Geometry check sheet. Reference: the model listing, model coordinates, mm. Coordinates: 2 decimals unless noted, no trailing zeros. Loops run counter-clockwise (first coordinate to the right, second up) from the corner with the lowest first, then second, coordinate; pieces in that order, holes last. Notation, with made-up numbers: (83, -25) -> (138, -25) arc R19 cw to (138, -14) -> close; hole circle Ø1 at (-23.5, 28). An arc over 180 degrees is marked (long way). Answer as a JSON object with one key per item and string values.
from build123d import *

# Parameters (mm, degrees)
F0_R     = 8
F1_DEPTH = 6
F4_DEPTH = 16.001
F5_R     = 20
F6_R     = 0.5


with BuildPart() as f1:
    # F0 (on Top) → F1 (new body)
    with BuildSketch(Plane.XY):
        Circle(F0_R)
    extrude(amount=F1_DEPTH)

    # F3 (on offset) → F4 (cut, through all)
    with BuildSketch(Plane.XZ.offset(8)):
        Polygon((8, 6), (-8, 6), (0, 4.4), align=None)
    extrude(amount=-F4_DEPTH, mode=Mode.SUBTRACT)

    # F5
    f5_edges = [f1.edges().sort_by_distance(p)[0] for p in [
        (0, 0, 4.4),
    ]]
    fillet(f5_edges, radius=F5_R)

    # F6
    f6_edges = [f1.edges().sort_by_distance(p)[0] for p in [
        (-6.896857, -4.053808, 5.779371),
        (-6.896857, 4.053808, 5.779371),
    ]]
    fillet(f6_edges, radius=F6_R)


solid = f1.part
1. Mould release check, pull along X, two halves, no side actions. Record for faces 1 (the face through (3.69, -7.1, 2.66)), 2 (the face through (-5.3, -0.09, 5.46)), 3 (the face through (0, 0, 0)): released by +X, released by -X, zero draft, split by the parting line, or undercut.
Evaluation:
{"face 1": "split by the parting line", "face 2": "undercut", "face 3": "zero draft"}
2. Depth check by flat-ended pin: P1, Ø1, axis at y = 3.5, z = 2, coming from the -X side; P2, Ø1.5, axis at x = -4.5, y = -3, coming from the -Z side; P3, Ø3, axis at x = -4.5, y = 2, coming from the +Z side; P4, Ø6, axis at x = -1, y = -3.5, coming from the +Z side. Enter the tip coordinate at first touch or a pass-through.
Evaluation:
{"P1": "stops at x = -7.42", "P2": "stops at z = 0", "P3": "stops at z = 5.6", "P4": "stops at z = 5.2"}
3. Thickness scan on probe 1 along X at (y, z) = (0.25, 2.3); probe 2 along Z at (x, y) = (3, 6); probe 3 along X at (y, z) = (7.25, 3.9). Record the ranges inside material, lowest first. Write a range as from..to.
Evaluation:
{"probe 1": "x = -8..8", "probe 2": "z = 0..5.02", "probe 3": "x = -3.38..3.38"}
4. Section check A-A, the plane z = 3.3. Record the boundary of the cut face in (x, y), then the cut area to 3 significant figures.
Evaluation:
{"outline": "circle Ø16 at (0, 0)", "area": "201 mm^2"}
